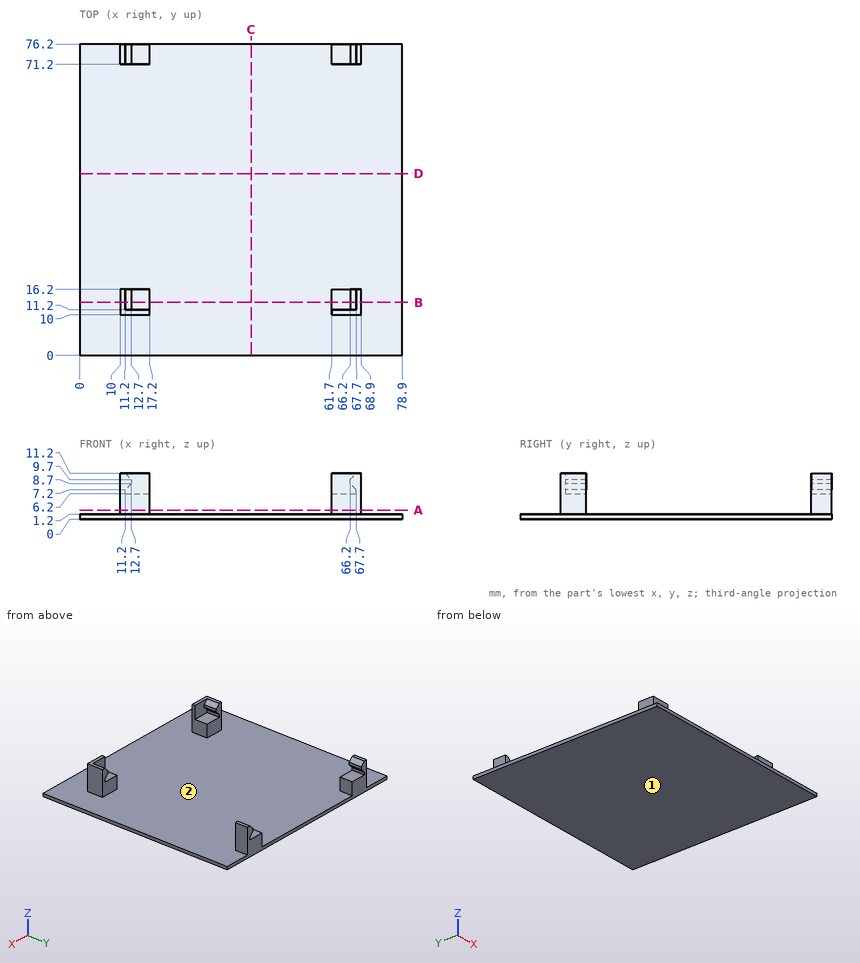
Job drawing, mm, ordinate dimensions from the low corner. One solid piece. Give positions to 0.01 mm unless a question says otherwise; leave off trailing zeros. Loops run counter-clockwise (first coordinate to the right, second up) from the corner with the lowest first, then second, coordinate; pieces in that order, holes last. Notation, with made-up numbers: M 56.5,82 L 84.5,82 A26 ccw 84.5,114 Z; hole C 43.25,-30.75 d9. An arc over 180 degrees is marked long. Return JSON: item names as keys, results as strings.
1) Flat gauge pins, fed straight in: pin 1 Ø1.5 at (x, y) = (62, 12.5) entering from +Z; pin 2 Ø1.5 at (y, z) = (74.5, 3) entering from -X; pin 3 Ø1.1 at (y, z) = (73, 6.5) entering from +X. Where does each tip first touch, or does it go through?
Calculated:
{"pin 1": "stops at z = 6.2", "pin 2": "stops at x = 10", "pin 3": "stops at x = 68.9"}
2) Saw through at D-D, the plane y = 44.5. List the corners of the cut face in (x, z).
Calculated:
{"outline": "M 0,0 L 78.9,0 L 78.9,1.2 L 0,1.2 Z"}
3) Saw through at C-C, the plane x = 42. List the corners of the cut face in (y, z), then the cut area to 3 significant figures.
Calculated:
{"outline": "M 0,0 L 76.2,0 L 76.2,1.2 L 0,1.2 Z", "area": "91.4 mm2"}
4) Saw through at A-A, the plane z = 2.25. List the corners of the cut face in (x, y), then the cut area to 3 significant figures.
Calculated:
{"outline": "M 10,10 L 17.2,10 L 17.2,16.2 L 10,16.2 Z; M 10,71.2 L 17.2,71.2 L 17.2,76.2 L 10,76.2 Z; M 61.7,10 L 68.9,10 L 68.9,16.2 L 61.7,16.2 Z; M 61.7,71.2 L 68.9,71.2 L 68.9,76.2 L 61.7,76.2 Z", "area": "161 mm2"}
5) Pull direction Y, two halves, no side cores. Call the marked faces 1 and 2: released by +Y, released by -Y, zero draft, split by the parting line, or undercut.
Calculated:
{"face 1": "zero draft", "face 2": "undercut"}
6) Drill centre lines: line 1 (Y direction, x = 63, z = 5.25); line 2 (Z direction, x = 20.5, y = 28); line 3 (Y direction, x = 62, z = 8.5). Where is each one in solid material? Low to high.
Calculated:
{"line 1": "y = 10 to 16.2, 71.2 to 76.2", "line 2": "z = 0 to 1.2", "line 3": "y = 10 to 11.2"}
7) Saw through at B-B, the plane y = 13. List the corners of the cut face in (x, z), then the cut area to 3 significant figures.
Calculated:
{"outline": "M 0,0 L 78.9,0 L 78.9,1.2 L 68.9,1.2 L 68.9,11.2 L 67.7,11.2 L 66.2,9.7 L 66.2,8.7 L 67.7,7.2 L 67.7,6.2 L 61.7,6.2 L 61.7,1.2 L 17.2,1.2 L 17.2,6.2 L 11.2,6.2 L 11.2,7.2 L 12.7,8.7 L 12.7,9.7 L 11.2,11.2 L 10,11.2 L 10,1.2 L 0,1.2 Z", "area": "186 mm2"}
